```python
from build123d import *

# Parameters (mm, degrees)
F0_W     = 180
F0_H     = 240
F1_DEPTH = 75
F3_D     = 10
F3_DEPTH = 600
F3_TIP   = 3.0043030951
F2_R     = 10
F2_R_2   = 5
F4_DEPTH = 15


with BuildPart() as f1:
    # F0 (on Front) → F1 (new body, symmetric)
    with BuildSketch(Plane.XZ):
        Polygon((387.4092161655, 284.3629608303), (187.4092161655, 284.3629608303), (187.4092161655, 34.3629608303), (-212.5907838345, 34.3629608303), (-212.5907838345, 24.3629608303), (787.4092161655, 24.3629608303), (787.4092161655, 34.3629608303), (387.4092161655, 34.3629608303), align=None)
        with Locations((287.4092161655, 154.3629608303)):
            Rectangle(F0_W, F0_H, mode=Mode.SUBTRACT)
    extrude(amount=F1_DEPTH, both=True)

    # F3 (one way)
    with BuildSketch(Plane.XY.offset(34.3629608303)):
        with Locations((287.4092161655, 0)):
            Circle(F3_D / 2)
    extrude(amount=-F3_DEPTH, mode=Mode.SUBTRACT)
    with Locations(Plane.XY.offset(34.3629608303)):
        with Locations((287.4092161655, 0)):
            with Locations((0, 0, -(F3_DEPTH + F3_TIP / 2))):  # 118° drill point
                Cone(0, F3_D / 2, F3_TIP, mode=Mode.SUBTRACT)

    # F2 (on face) → F4 (join)
    with BuildSketch(Plane.XY.offset(34.3629608303)):
        with Locations((287.4092161655, 0)):
            Circle(F2_R)
        with Locations((287.4092161655, 0)):
            Circle(F2_R_2, mode=Mode.SUBTRACT)
    extrude(amount=F4_DEPTH)


solid = f1.part
```
Can you work these out from the model? Positions are in its coordinate system, mm. A direction names the side the tool comes from. Give positions to 0.01 mm unless a question says otherwise; leave off trailing zeros. Order: outer loops, then holes, each group sorted by start corner. A loop starts at its lowest first (then second) coordinate and runs counter-clockwise, first axis right, second up. Notation, with made-up numbers: M -38,51 L -22,51 A24 cw -22,79 Z; hole C -29,63 d2. An arc over 180 degrees is marked long. One line per item, written item: value.
1) I want a section at B-B, the plane z = 168. List the corners of the cut face in (x, y) for me.
Answer sheet:
outline: M 187.41,-75 L 197.41,-75 L 197.41,75 L 187.41,75 Z; M 377.41,-75 L 387.41,-75 L 387.41,75 L 377.41,75 Z
2) We'd pull the mould along Z, two halves only. Please class faces 1 (the face through (-10, -1, 34.363)), 2 (the face through (285, 75, 30)), 3 (the face through (280, -1, 24.363)), 4 (the face through (197.409, -1, 153)): released by +Z, released by -Z, zero draft, split by the parting line, or undercut.
Answer sheet:
face 1: released by +Z
face 2: zero draft
face 3: released by -Z
face 4: undercut
3) On a 3-axis mill with a long thin cutter (end or side, diameter ignored), from which of +Z, -Z, +X, -X, +Y, -Y can I reach the whole of each face in a straight line? I mean faces 5 (the face through (289, 5, 49.363)), 6 (the face through (277.42, 0.44, 41.76)), 7 (the face through (387.409, -1, 158)). Say none if no direction works.
Answer sheet:
face 5: +Y, -Y
face 6: none
face 7: +Z, +X, +Y, -Y
4) I want a section at A-A, the plane x = 235. List the corners of the cut face in (y, z) for me.
Answer sheet:
outline: M -75,24.36 L 75,24.36 L 75,34.36 L -75,34.36 Z; M -75,274.36 L 75,274.36 L 75,284.36 L -75,284.36 Z
5) Please list where these lines run through material, in increasing order: line 1 along X through (y, z) = (-67.5, 221); line 2 along Z through (x, y) = (299.5, 18.5); line 3 along Z through (x, y) = (732, -68).
Answer sheet:
line 1: x = 187.41 to 197.41, 377.41 to 387.41
line 2: z = 24.36 to 34.36, 274.36 to 284.36
line 3: z = 24.36 to 34.36
6) I want a section at C-C, the plane y = -24.5. List the corners of the cut face in (x, z) for me.
Answer sheet:
outline: M -212.59,24.36 L 787.41,24.36 L 787.41,34.36 L 387.41,34.36 L 387.41,284.36 L 187.41,284.36 L 187.41,34.36 L -212.59,34.36 Z; hole M 197.41,34.36 L 377.41,34.36 L 377.41,274.36 L 197.41,274.36 Z
7) I want a section at D-D, the plane x = 551. List the corners of the cut face in (y, z) for me.
Answer sheet:
outline: M -75,24.36 L 75,24.36 L 75,34.36 L -75,34.36 Z
8) For P1, Ø6, axis at y = -28.5, z = 63, coming from the +X side; P2, Ø1.5, axis at x = 562.5, y = 21.5, coming from the +Z side; P3, Ø8, axis at y = -12, z = 74.5, coming from the -X side, each with a flat end and sliding along its axis, tell me the tip position at first contact or that it passes through.
Answer sheet:
P1: stops at x = 387.41
P2: stops at z = 34.36
P3: stops at x = 187.41
